CAD build for the part. Positions are in the model's coordinates, mm. Give positions to 0.01 mm unless a question says otherwise; leave off trailing zeros. Loops run counter-clockwise (first coordinate to the right, second up) from the corner with the lowest first, then second, coordinate; pieces in that order, holes last. Notation, with made-up numbers: (18.25, -30.75) -> (69.25, -30.75) arc R16 cw to (69.25, -3.75) -> close; hole circle Ø7 at (1, 77.5). An arc over 180 degrees is marked (long way). Write each question's results on one line, items separated by ' | '. Start each with the question number.
```python
from build123d import *

# Parameters (mm, degrees)
SKIZZE1_W                       = 76
SKIZZE1_H                       = 12
AUFSATZ_LINEAR_AUSTRAGEN1_DEPTH = 5
VERRUNDUNG1_R                   = 6
F_6_0_6_DURCHMESSER_BOHRUNG3_D  = 6


with BuildPart() as part:
    # Skizze1 → Aufsatz-Linear austragen1 (new body)
    with BuildSketch(Plane.XY):
        Rectangle(SKIZZE1_W, SKIZZE1_H)
    extrude(amount=AUFSATZ_LINEAR_AUSTRAGEN1_DEPTH)

    # Verrundung1
    verrundung1_edges = [part.edges().sort_by_distance(p)[0] for p in [
        (-38, -6, 2.5),
        (38, -6, 2.5),
        (38, 6, 2.5),
        (-38, 6, 2.5),
    ]]
    fillet(verrundung1_edges, radius=VERRUNDUNG1_R - 0.0001)  # a hair under: the kernel refuses the full size

    # Ø6.0 (6) Durchmesser Bohrung3 (through all)
    with Locations(Plane.XY.offset(5)):
        with Locations((-32, 0), (32, 0)):
            Hole(F_6_0_6_DURCHMESSER_BOHRUNG3_D / 2)


solid = part.part
```
Q1. Mould opens along Z. For faces 1 (the face through (36.196, -4.289, 2.535)), 2 (the face through (-1, 0, 0)), 3 (the face through (-1, 0, 5)) say: pulls with the +Z half, pulls with the -Z half, needs draft (parallel to the pull), parting line crosses it, or undercut.
Q2. Saw through at B-B, the plane y = 1. List the corners of the cut face in (x, z), then the cut area to 3 significant figures.
Q3. Wall check: L1, parallel to Y at x = 32, z = 3.45; L2, parallel to X at y = -2, z = 4.35; L3, parallel to X at y = 1.25, z = 4.1. Give the ranges that are in metal, low to high.
Q4. Drop flat-ended pins along their axis: pin 1 (2 mm diameter, centred on y = 0.5, z = 4, fed in from -X); pin 2 (3.5 mm diameter, centred on x = -32, y = 0, fed in from -Z); pin 3 (2 mm diameter, centred on y = -4.5, z = 1.5, fed in from -X). Give the stop position or say it passes through.
Q5. Saw through at A-A, the plane z = 3.35. Give the number of separate pieces and of enclosed holes in the cut face, then the cut area to 3 significant figures.
Answer block:
1) face 1: needs draft | face 2: pulls with the -Z half | face 3: pulls with the +Z half
2) outline: (-37.92, 0) -> (-34.83, 0) -> (-34.83, 5) -> (-37.92, 5) -> close; (-29.17, 0) -> (29.17, 0) -> (29.17, 5) -> (-29.17, 5) -> close; (34.83, 0) -> (37.92, 0) -> (37.92, 5) -> (34.83, 5) -> close | area: 323 mm2
3) L1: y = -6 to -3, 3 to 6 | L2: x = -37.66 to -34.24, -29.76 to 29.76, 34.24 to 37.66 | L3: x = -37.87 to -34.73, -29.27 to 29.27, 34.73 to 37.87
4) pin 1: stops at x = -38 | pin 2: passes through | pin 3: stops at x = -36.87
5) separate pieces: 1 | enclosed holes: 2 | area: 825 mm2
